Verification items for the finished model (mm, model axes). Face numbers are marked on the shaded views. A direction names the side the tool comes from. Give positions to 0.01 mm unless a question says otherwise; leave off trailing zeros. Write each loop counter-clockwise with the first axis right and the second up, starting at its lowest first coordinate (ties: lowest second). Pieces come first, ordered by that corner, then holes. Notation, with made-up numbers: (-4.75, 54.5) -> (50.25, 54.5) arc R19 cw to (50.25, 73.5) -> close; hole circle Ø5 at (-37.5, 49). An arc over 180 degrees is marked (long way). Answer as CSV lines item,"result". Start each with the question number.
1) Sectioned sample at A-A on z = 0. Record the cut outline in (x, y), and give its area (3 significant figures).
2) Tool access check on the marked faces 1, 2, 3, 4 and 5. Record the directions out of +Z, -Z, +X, -X, +Y, -Y that give a thin tool (end or side, any length) a straight path to the whole face; none if there is none.
3) Sectioned sample at B-B on x = 8. Record the cut outline in (y, z).
4) Sectioned sample at D-D on z = -6.5. Record the cut outline in (x, y).
5) Sectioned sample at C-C on y = 11.5. Record the cut outline in (x, z).
6) Material ranges on L1, parallel to X at y = 9.5, z = 0; L2, parallel to X at y = 3.5, z = 0; L3, parallel to X at y = 11, z = -2, recorded low to high.
7) Mould release check, pull along Z, two halves, no side actions. Record for the marked faces 6, 7 and 8: released by +Z, released by -Z, zero draft, split by the parting line, or undercut.
8) Gauge pin test, flat ends, axial feed: pin 1 Ø2 at (x, y) = (0.5, 10.5) entering from -Z; pin 2 Ø6 at (y, z) = (3.5, -5.5) entering from -X; pin 3 Ø4 at (x, z) = (16, -17) entering from +Y; pin 4 Ø24 at (x, z) = (9, -9.5) entering from +Y. Record the tip position at first contact, or that the pin passes through.
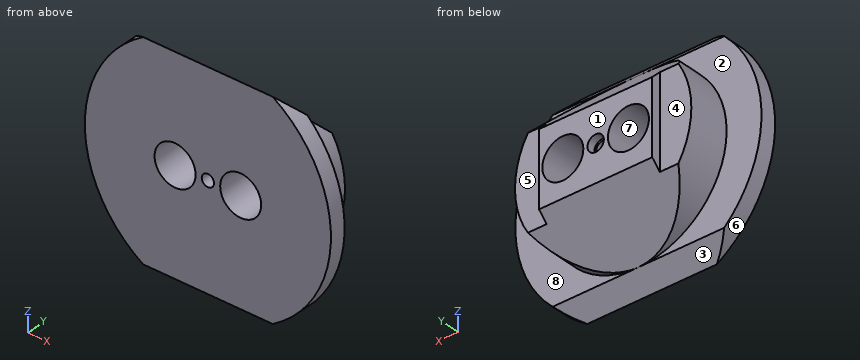
```python
from build123d import *
from build123d.topology import SkipClean

# Parameters (mm, degrees)
SKETCH1_R                            = 30
BOSS_EXTRUDE1_DEPTH                  = 4
BOSS_EXTRUDE2_REACH                  = 44.615
BOSS_EXTRUDE2_END_RADIUS             = 30
BOSS_EXTRUDE2_DIRECTION_2_REACH      = 44.615
BOSS_EXTRUDE2_DIRECTION_2_END_RADIUS = 30
SKETCH3_OUTSIDE_W                    = 78.092
SKETCH3_OUTSIDE_H                    = 69.092
SKETCH3_OUTSIDE_R                    = 21.5
CUT_EXTRUDE2_DEPTH                   = 12.5
BOSS_EXTRUDE3_DEPTH                  = 18
BOSS_EXTRUDE4_DEPTH                  = 15
BOSS_EXTRUDE5_DEPTH                  = 15
CUT_EXTRUDE3_DEPTH                   = 44.292609069
CUT_EXTRUDE3_DEPTH_BACK              = 44.292609069
SKETCH8_R                            = 2
CUT_EXTRUDE8_DEPTH                   = 48.077064479
CUT_EXTRUDE8_DEPTH_BACK              = 48.077064479
CUT_EXTRUDE9_DEPTH                   = 59.659818207
CUT_EXTRUDE11_DEPTH                  = 20
CUT_EXTRUDE12_DEPTH                  = 20
CUT_EXTRUDE13_DEPTH                  = 20
CUT_EXTRUDE14_DEPTH                  = 44.292609069
CUT_EXTRUDE14_DEPTH_BACK             = 44.292609069
SKETCH25_W                           = 66.075437062
SKETCH25_H                           = 20.142243048
SKETCH26_R                           = 5
CUT_EXTRUDE15_DEPTH                  = 24
CUT_EXTRUDE17_DEPTH                  = 47.524187258
CUT_EXTRUDE17_DEPTH_BACK             = 47.524187258
SKETCH29_W                           = 7.7
SKETCH29_H                           = 2.2
CUT_EXTRUDE18_DEPTH                  = 47.524187258
CUT_EXTRUDE18_DEPTH_BACK             = 47.524187258
SKETCH31_W                           = 7.7
SKETCH31_H                           = 2.2
SKETCH34_R                           = 1.5
CUT_EXTRUDE21_DEPTH                  = 20
SKETCH35_R                           = 2
CUT_EXTRUDE22_DEPTH                  = 2


with BuildPart() as part:
    # Sketch1 → Boss-Extrude1 (new body)
    with BuildSketch(Plane(origin=(0, 0, 0), x_dir=(1, 0, 0), z_dir=(0, 1, 0))):
        with Locations(Location((0, 0, 0), (0, 0, 270))):
            Circle(SKETCH1_R)
    extrude(amount=BOSS_EXTRUDE1_DEPTH)

    # Boss-Extrude2: up to this cylinder (the profile starts inside it)
    with SkipClean():  # the faces are left unmerged after this step: merging them gives an invalid solid
        boss_extrude2_end = Plane(origin=(0, 9.396175, 0), z_dir=(0, -1, 0)) * Cylinder(BOSS_EXTRUDE2_END_RADIUS, 150.23, mode=Mode.PRIVATE)
        # Sketch2 → Boss-Extrude2 (add, up to the surface)
        with BuildSketch(Plane(origin=(0, 0, 0), x_dir=(0, 0, -1), z_dir=(1, 0, 0)), mode=Mode.PRIVATE) as boss_extrude2_sk1:
            Polygon((0, 4), (21.5, 4), (9, 16.5), (-9, 16.5), (-21.5, 4), align=None)
        boss_extrude2_tool1 = extrude(boss_extrude2_sk1.sketch, amount=BOSS_EXTRUDE2_REACH, mode=Mode.PRIVATE) & boss_extrude2_end
        add(boss_extrude2_tool1.solids().sort_by_distance((0, 9.396175, 0))[0])

    # Boss-Extrude2 direction 2: up to this cylinder (the profile starts inside it)
    with SkipClean():  # the faces are left unmerged after this step: merging them gives an invalid solid
        boss_extrude2_direction_2_end = Plane(origin=(0, 9.396175, 0), z_dir=(0, -1, 0)) * Cylinder(BOSS_EXTRUDE2_DIRECTION_2_END_RADIUS, 150.23, mode=Mode.PRIVATE)
        # Sketch2 → Boss-Extrude2 direction 2 (add, up to the surface)
        with BuildSketch(Plane(origin=(0, 0, 0), x_dir=(0, 0, -1), z_dir=(1, 0, 0)), mode=Mode.PRIVATE) as boss_extrude2_direction_2_sk1:
            Polygon((0, 4), (21.5, 4), (9, 16.5), (-9, 16.5), (-21.5, 4), align=None)
        boss_extrude2_direction_2_tool1 = extrude(boss_extrude2_direction_2_sk1.sketch, amount=-BOSS_EXTRUDE2_DIRECTION_2_REACH, mode=Mode.PRIVATE) & boss_extrude2_direction_2_end
        add(boss_extrude2_direction_2_tool1.solids().sort_by_distance((0, 9.396175, 0))[0])

    # SurfaceCut1
    split(bisect_by=Plane(origin=(0, 12.75, -12.75), x_dir=(1, 0, 0), z_dir=(0, 0.7071067811865558, -0.7071067811865392)), keep=Keep.BOTTOM)

    # SurfaceCut2
    split(bisect_by=Plane(origin=(0, 12.75, 12.75), x_dir=(1, 0, 0), z_dir=(0, 0.7071067811865509, 0.7071067811865442)), keep=Keep.BOTTOM)

    # Sketch3 outside → Cut-Extrude2 (cut)
    with BuildSketch(Plane(origin=(0, 4, 0), x_dir=(1, 0, 0), z_dir=(0, 1, 0))):
        Rectangle(SKETCH3_OUTSIDE_W, SKETCH3_OUTSIDE_H)
        Circle(SKETCH3_OUTSIDE_R, mode=Mode.SUBTRACT)
    extrude(amount=CUT_EXTRUDE2_DEPTH, mode=Mode.SUBTRACT)

    # Sketch5 → Boss-Extrude3 (add)
    with BuildSketch(Plane(origin=(0, 0, 0), x_dir=(-1, 0, 0), z_dir=(0, -1, 0))):
        Polygon((0, -6), (-17.5, -6), (-17.5, 6), (17.5, 6), (17.5, -6), align=None)
    extrude(amount=BOSS_EXTRUDE3_DEPTH)

    # Sketch6 → Boss-Extrude4 (add)
    with BuildSketch(Plane.XZ):
        Polygon((0, 15), (7, 15), (7, 6), (-7, 6), (-7, 15), align=None)
    extrude(amount=BOSS_EXTRUDE4_DEPTH)

    # Sketch7 → Boss-Extrude5 (add)
    with BuildSketch(Plane.XZ):
        Polygon((0, -15), (7, -15), (7, -6), (-7, -6), (-7, -15), align=None)
    extrude(amount=BOSS_EXTRUDE5_DEPTH)

    # Sketch8 → Cut-Extrude3 (cut, two sides: drawn at the far end of the back side and taken through both)
    with BuildSketch(Plane.XY.offset(-CUT_EXTRUDE3_DEPTH_BACK)):
        with Locations((-12.5, -12.5)):
            Circle(SKETCH8_R)
        with Locations((12.5, -12.5)):
            Circle(SKETCH8_R)
    extrude(amount=CUT_EXTRUDE3_DEPTH + CUT_EXTRUDE3_DEPTH_BACK, mode=Mode.SUBTRACT)

    # Sketch16 → Cut-Extrude8 (cut, two sides: drawn at the far end of the back side and taken through both)
    with BuildSketch(Plane.XY.offset(6).offset(-CUT_EXTRUDE8_DEPTH_BACK)):
        Polygon((17.5, -18), (17.5, -14.5), (14, -18), align=None)
        Polygon((-17.5, -18), (-14, -18), (-17.5, -14.5), align=None)
    extrude(amount=CUT_EXTRUDE8_DEPTH + CUT_EXTRUDE8_DEPTH_BACK, mode=Mode.SUBTRACT)

    # Sketch17 → Cut-Extrude9 (cut, through all)
    with BuildSketch(Plane(origin=(10.365975269, -9.674910251, -8.062425209), x_dir=(-0.3613483622370374, 0.337258471421235, -0.8693009171531012), z_dir=(0.6355070151731325, -0.5931398808282571, -0.49428323402354774))):
        Polygon((-2.372510104, -6.189601271), (7.980636686, -0.706686759), (7.980636686, -10.965829024), align=None)
    extrude(amount=CUT_EXTRUDE9_DEPTH, mode=Mode.SUBTRACT)

    # Sketch19 → Cut-Extrude11 (cut)
    with BuildSketch(Plane(origin=(-10.365975269, -9.674910251, -8.062425209), x_dir=(0.3613483622370374, 0.33725847142123494, -0.8693009171531012), z_dir=(0.6355070151731324, 0.5931398808282571, 0.4942832340235476))):
        Polygon((-2.372510104, -6.189601271), (7.980636686, -10.965829024), (7.980636686, -0.706686759), align=None)
    extrude(amount=-CUT_EXTRUDE11_DEPTH, mode=Mode.SUBTRACT)

    # Sketch20 → Cut-Extrude12 (cut)
    with BuildSketch(Plane(origin=(-10.365975269, -9.674910251, 8.062425209), x_dir=(-0.3613483622370374, -0.3372584714212349, -0.8693009171531013), z_dir=(0.6355070151731326, 0.593139880828257, -0.49428323402354757))):
        Polygon((2.372510104, -6.189601271), (-7.980636686, -0.706686759), (-7.980636686, -10.965829024), align=None)
    extrude(amount=-CUT_EXTRUDE12_DEPTH, mode=Mode.SUBTRACT)

    # Sketch21 → Cut-Extrude13 (cut)
    with BuildSketch(Plane(origin=(10.365975269, -9.674910251, 8.062425209), x_dir=(-0.3613483622370374, 0.3372584714212349, 0.8693009171531013), z_dir=(-0.6355070151731326, 0.593139880828257, -0.49428323402354757))):
        Polygon((-2.372510104, -6.189601271), (7.980636686, -0.706686759), (7.980636686, -10.965829024), align=None)
    extrude(amount=-CUT_EXTRUDE13_DEPTH, mode=Mode.SUBTRACT)

    # Sketch25 → Cut-Extrude14 (cut, two sides: drawn at the far end of the back side and taken through both)
    with BuildSketch(Plane.XY.offset(-CUT_EXTRUDE14_DEPTH_BACK)):
        with Locations((0, -10.071121524)):
            Rectangle(SKETCH25_W, SKETCH25_H)
    extrude(amount=CUT_EXTRUDE14_DEPTH + CUT_EXTRUDE14_DEPTH_BACK, mode=Mode.SUBTRACT)

    # Sketch26 → Cut-Extrude15 (cut)
    with BuildSketch(Plane(origin=(0, 16.5, 0), x_dir=(1, 0, 0), z_dir=(0, 1, 0))):
        with Locations(Location((-8, 0, 0), (0, 0, 270))):
            Circle(SKETCH26_R)
        with Locations(Location((8, 0, 0), (0, 0, 270))):
            Circle(SKETCH26_R)
    extrude(amount=-CUT_EXTRUDE15_DEPTH, mode=Mode.SUBTRACT)

    # Sketch29 → Cut-Extrude17 (cut, two sides: drawn at the far end of the back side and taken through both)
    with BuildSketch(Plane.XY.offset(6).offset(-CUT_EXTRUDE17_DEPTH_BACK)):
        with Locations((17.65, 15.4)):
            Rectangle(SKETCH29_W, SKETCH29_H)
    extrude(amount=CUT_EXTRUDE17_DEPTH + CUT_EXTRUDE17_DEPTH_BACK, mode=Mode.SUBTRACT)

    # Sketch31 → Cut-Extrude18 (cut, two sides: drawn at the far end of the back side and taken through both)
    with BuildSketch(Plane.XY.offset(6).offset(-CUT_EXTRUDE18_DEPTH_BACK)):
        with Locations((-17.65, 15.4)):
            Rectangle(SKETCH31_W, SKETCH31_H)
    extrude(amount=CUT_EXTRUDE18_DEPTH + CUT_EXTRUDE18_DEPTH_BACK, mode=Mode.SUBTRACT)

    # Sketch34 → Cut-Extrude21 (cut)
    with BuildSketch(Plane.XZ):
        with Locations(Location((0, 0, 0), (0, 0, 270))):
            Circle(SKETCH34_R)
    extrude(amount=-CUT_EXTRUDE21_DEPTH, mode=Mode.SUBTRACT)

    # Sketch35 → Cut-Extrude22 (cut)
    with BuildSketch(Plane(origin=(0, 16.5, 0), x_dir=(1, 0, 0), z_dir=(0, 1, 0))):
        with Locations(Location((0, 0, 0), (0, 0, 270))):
            Circle(SKETCH35_R)
    extrude(amount=-CUT_EXTRUDE22_DEPTH, mode=Mode.SUBTRACT)


solid = part.part
```
Ans:
1,outline,"(-30, 0) -> (-13, 0) -> (-13, 16.5) -> (-13.8, 16.5) -> (-13.8, 14.3) -> (-21.5, 14.3) -> (-21.5, 4) -> (-30, 4) -> close; (-3, 0) -> (-1.5, 0) -> (-1.5, 14.5) -> (-2, 14.5) -> (-2, 16.5) -> (-3, 16.5) -> close; (1.5, 0) -> (3, 0) -> (3, 16.5) -> (2, 16.5) -> (2, 14.5) -> (1.5, 14.5) -> close; (13, 0) -> (30, 0) -> (30, 4) -> (21.5, 4) -> (21.5, 14.3) -> (13.8, 14.3) -> (13.8, 16.5) -> (13, 16.5) -> close"
1,area,"362 mm²"
2,face 1,"+Z, -Z, +X, -X, +Y"
2,face 2,"-X, +Y"
2,face 3,"-Z, +X, -X, +Y"
2,face 4,"+Z, -Z, -X, +Y"
2,face 5,"+Z, -Z, +X, +Y"
3,outline,"(0, -25.5) -> (4, -21.5) -> (4, -19.96) -> (5.54, -19.96) -> (16.5, -9) -> (16.5, -5) -> (0, -5) -> close; (0, 5) -> (16.5, 5) -> (16.5, 9) -> (5.54, 19.96) -> (4, 19.96) -> (4, 21.5) -> (0, 25.5) -> close"
4,outline,"(-29.29, 0) -> (29.29, 0) -> (29.29, 4) -> (20.49, 4) -> (20.49, 14.3) -> (13.8, 14.3) -> (13.8, 16.5) -> (-13.8, 16.5) -> (-13.8, 14.3) -> (-20.49, 14.3) -> (-20.49, 4) -> (-29.29, 4) -> close"
5,outline,"(-16.32, -14) -> (16.32, -14) arc R21.5 ccw to (16.32, 14) -> (-16.32, 14) arc R21.5 ccw to start; hole circle Ø10 at (-8, 0); hole circle Ø3 at (0, 0); hole circle Ø10 at (8, 0)"
6,L1,"x = -21.5 to -13, -3 to -1.5, 1.5 to 3, 13 to 21.5"
6,L2,"x = -30 to -13, -3 to -1.5, 1.5 to 3, 13 to 30"
6,L3,"x = -21.41 to -12.58, -3.42 to 3.42, 12.58 to 21.41"
7,face 6,"split by the parting line"
7,face 7,"undercut"
7,face 8,"zero draft"
8,pin 1,"stops at z = -16"
8,pin 2,"stops at x = -29.9"
8,pin 3,"stops at y = 10.36"
8,pin 4,"stops at y = 16.5"
